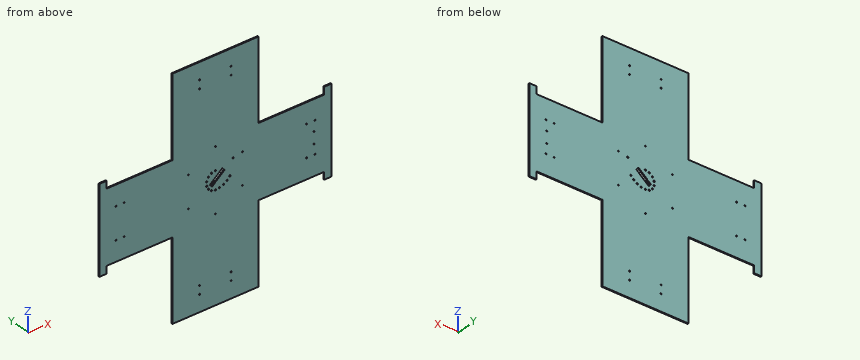
from build123d import *

# Parameters (mm, degrees)
BOSS_EXTRUDE1_DEPTH = 3
SKETCH2_R           = 1.6
CUT_EXTRUDE1_DEPTH  = 495.98383812
SKETCH3_R           = 2
SKETCH3_R_2         = 1.5
CUT_EXTRUDE2_DEPTH  = 495.98383812


with BuildPart() as part:
    # Sketch1 → Boss-Extrude1 (new body)
    with BuildSketch(Plane(origin=(0, 0, 0), x_dir=(1, 0, 0), z_dir=(0, 1, 0))):
        Polygon((-350, -130), (-328, -130), (-328, -108), (-130, -108), (-130, -130), (-130, -350), (130, -350), (130, -130), (130, -108), (328, -108), (328, -130), (350, -130), (350, 130), (328, 130), (328, 108), (130, 108), (130, 130), (130, 350), (-130, 350), (-130, 130), (-130, 108), (-328, 108), (-328, 130), (-350, 130), align=None)
    extrude(amount=BOSS_EXTRUDE1_DEPTH)

    # Sketch2 → Cut-Extrude1 (cut, through all)
    with BuildSketch(Plane(origin=(0, 3, 0), x_dir=(1, 0, 0), z_dir=(0, 1, 0))):
        with Locations(Location((-300, 47.5, 0), (0, 0, 270))):
            Circle(SKETCH2_R)
        with Locations(Location((-300, -47.5, 0), (0, 0, 270))):
            Circle(SKETCH2_R)
        with Locations(Location((-47.5, 300, 0), (0, 0, 270))):
            Circle(SKETCH2_R)
        with Locations(Location((47.5, 300, 0), (0, 0, 270))):
            Circle(SKETCH2_R)
        with Locations(Location((-47.5, -300, 0), (0, 0, 270))):
            Circle(SKETCH2_R)
        with Locations(Location((47.5, -300, 0), (0, 0, 270))):
            Circle(SKETCH2_R)
        with Locations(Location((300, 47.5, 0), (0, 0, 270))):
            Circle(SKETCH2_R)
        with Locations(Location((300, -47.5, 0), (0, 0, 270))):
            Circle(SKETCH2_R)
        with Locations(Location((-275, 47.5, 0), (0, 0, 270))):
            Circle(SKETCH2_R)
        with Locations(Location((-275, -47.5, 0), (0, 0, 270))):
            Circle(SKETCH2_R)
        with Locations(Location((-47.5, 275, 0), (0, 0, 270))):
            Circle(SKETCH2_R)
        with Locations(Location((47.5, 275, 0), (0, 0, 270))):
            Circle(SKETCH2_R)
        with Locations(Location((275, 47.5, 0), (0, 0, 270))):
            Circle(SKETCH2_R)
        with Locations(Location((275, -47.5, 0), (0, 0, 270))):
            Circle(SKETCH2_R)
        with Locations(Location((-47.5, -275, 0), (0, 0, 270))):
            Circle(SKETCH2_R)
        with Locations(Location((47.5, -275, 0), (0, 0, 270))):
            Circle(SKETCH2_R)
        with Locations(Location((297.5, 17.5, 0), (0, 0, 270))):
            Circle(SKETCH2_R)
        with Locations(Location((297.5, -17.5, 0), (0, 0, 270))):
            Circle(SKETCH2_R)
    extrude(amount=-CUT_EXTRUDE1_DEPTH, mode=Mode.SUBTRACT)

    # Sketch3 → Cut-Extrude2 (cut, through all)
    with BuildSketch(Plane(origin=(0, 3, 0), x_dir=(1, 0, 0), z_dir=(0, 1, 0))):
        with Locations(Location((0, 27, 0), (0, 0, 270))):
            Circle(SKETCH3_R)
        with Locations(Location((12.537623126, 25.500271023, 0), (0, 0, 270))):
            Circle(SKETCH3_R)
        with Locations(Location((24.394492834, 21.157941995, 0), (0, 0, 270))):
            Circle(SKETCH3_R)
        with Locations(Location((34.951700365, 14.230709518, 0), (0, 0, 270))):
            Circle(SKETCH3_R)
        with Locations(Location((43.654980033, 5.082261362, 0), (0, 0, 270))):
            Circle(SKETCH3_R)
        with Locations(Location((53.119734703, -41.583325675, 0), (0, 0, 270))):
            Circle(SKETCH3_R)
        with Locations(Location((-11.667858187, 24.348738886, 0), (0, 0, 270))):
            Circle(SKETCH3_R)
        with Locations(Location((-21.089928763, 16.858674467, 0), (0, 0, 270))):
            Circle(SKETCH3_R)
        with Locations(Location((-26.320730998, 6.018232276, 0), (0, 0, 270))):
            Circle(SKETCH3_R)
        with Locations(Location((-26.320730998, -6.018232276, 0), (0, 0, 270))):
            Circle(SKETCH3_R)
        with Locations(Location((-21.089928763, -16.858674467, 0), (0, 0, 270))):
            Circle(SKETCH3_R)
        with Locations(Location((-11.667858187, -24.348738886, 0), (0, 0, 270))):
            Circle(SKETCH3_R)
        with Locations(Location((0.0730028, -26.999901307, 0), (0, 0, 270))):
            Circle(SKETCH3_R)
        with Locations(Location((0, 94.25, 0), (0, 0, 270))):
            Circle(SKETCH3_R_2)
        with Locations(Location((81.622894307, 47.125, 0), (0, 0, 270))):
            Circle(SKETCH3_R_2)
        with Locations(Location((81.622894307, -47.125, 0), (0, 0, 270))):
            Circle(SKETCH3_R_2)
        with Locations(Location((0, -94.25, 0), (0, 0, 270))):
            Circle(SKETCH3_R_2)
        with Locations(Location((-81.622894307, -47.125, 0), (0, 0, 270))):
            Circle(SKETCH3_R_2)
        with Locations(Location((-81.622894307, 47.125, 0), (0, 0, 270))):
            Circle(SKETCH3_R_2)
        Polygon((-5.400270308, -3.253491064), (20.858357141, -25.630588384), (27.47419461, -17.867168094), (1.21556716, 4.509929225), align=None)
        Polygon((-7.683629217, -1.307656515), (-5.737794668, 0.975702394), (-14.871230302, 8.759040592), (-16.817064852, 6.475681684), align=None)
        Polygon((-3.013626298, 4.172404866), (-1.067791749, 6.455763775), (-10.201227383, 14.239101973), (-12.147061933, 11.955743064), align=None)
    extrude(amount=-CUT_EXTRUDE2_DEPTH, mode=Mode.SUBTRACT)


solid = part.part
The listing builds one solid part. Answer for the finished solid, in the listing's coordinates (mm). Give positions to 0.01 mm unless a question says otherwise; leave off trailing zeros. Write each loop counter-clockwise with the first axis right and the second up, starting at its lowest first coordinate (ties: lowest second). Pieces come first, ordered by that corner, then holes. Notation, with made-up numbers: (38, 84.5) - (64, 84.5) arc R35 ccw to (64, 116.5) - close; hole circle Ø2 at (-1.5, -6). An arc over 180 degrees is marked (long way). One line per question, with ' | ' between items. Start each with the question number.
1. Straight lines are drawn through the part: line 1 (X direction, y = 1.65, z = -300); line 2 (X direction, y = 2.6, z = 17.5); line 3 (X direction, y = 2.35, z = 182). For each, find the intervals that lie inside material, in ascending order.
2. Section C-C, the plane y = 2.45 is taken. Count the separate pieces of the cut face and the enclosed holes in it, then the cut area to 3 significant figures.
3. Section B-B, the plane z = 182 is taken. Determine the outline of the cut face in (x, y).
4. Given P1, Ø3.5, axis at x = -300, z = -47.5, coming from the +Y side; P2, Ø0.9, axis at x = -251, y = 2, coming from the -Z side, each flat-ended and moving along its own axis, determine where each tip first touches the part or whether it passes through.
5. Section A-A, the plane x = 139 is taken. Determine the outline of the cut face in (y, z).
Result:
1) line 1: x = -130 to -49.1, -45.9 to 45.9, 49.1 to 130 | line 2: x = -350 to -22.98, -19.2 to 11.32, 27.04 to 295.9, 299.1 to 350 | line 3: x = -130 to 130
2) separate pieces: 1 | enclosed holes: 40 | area: 278,000 mm2
3) outline: (-130, 0) - (130, 0) - (130, 3) - (-130, 3) - close
4) P1: stops at y = 3 | P2: stops at z = -108
5) outline: (0, -108) - (3, -108) - (3, 108) - (0, 108) - close
